```python
from build123d import *

# Parameters (mm, degrees)
SKETCH1_R      = 3.3274
EXTRUDE1_DEPTH = 152.4


with BuildPart() as part:
    # Sketch1 → Extrude1 (new body)
    with BuildSketch(Plane.XY):
        with BuildLine():
            Line((-10.022898969, 12.91475973), (-5.252158105, 8.144007132))
            ThreePointArc((-5.252158105, 8.144007132), (-3.715177372, 7.117027388), (-1.902183975, 6.7564))
            Line((-1.902183975, 6.7564), (1.902183975, 6.7564))
            ThreePointArc((1.902183975, 6.7564), (3.715177372, 7.117027388), (5.252158105, 8.144007132))
            Line((5.252158105, 8.144007132), (10.022898969, 12.91475973))
            ThreePointArc((10.022898969, 12.91475973), (10.218362387, 13.207291992), (10.287, 13.552357131))
            Line((10.287, 13.552357131), (10.287, 14.0843))
            ThreePointArc((10.287, 14.0843), (10.022898185, 14.721898185), (9.3853, 14.986))
            Line((9.3853, 14.986), (5.617617549, 14.986))
            ThreePointArc((5.617617549, 14.986), (4.519044045, 15.441044045), (4.064, 16.539617549))
            Line((4.064, 16.539617549), (4.064, 17.496382451))
            ThreePointArc((4.064, 17.496382451), (4.519044045, 18.594955955), (5.617617549, 19.05))
            Line((5.617617549, 19.05), (7.974178704, 19.05))
            ThreePointArc((7.974178704, 19.05), (8.736178704, 18.288), (9.498178704, 19.05))
            Line((9.498178704, 19.05), (14.327719207, 19.05))
            ThreePointArc((14.327719207, 19.05), (15.087603123, 18.231251131), (15.847487039, 19.05))
            ThreePointArc((15.847487039, 19.05), (18.120176289, 18.120192083), (19.05, 15.847509295))
            ThreePointArc((19.05, 15.847509295), (18.231250992, 15.08762539), (19.05, 14.327741484))
            Line((19.05, 14.327741484), (19.05, 9.496091471))
            ThreePointArc((19.05, 9.496091471), (18.231250992, 8.736207565), (19.05, 7.97632366))
            Line((19.05, 7.97632366), (19.05, 5.617617549))
            ThreePointArc((19.05, 5.617617549), (18.594955955, 4.519044045), (17.496382451, 4.064))
            Line((17.496382451, 4.064), (16.539617549, 4.064))
            ThreePointArc((16.539617549, 4.064), (15.441044045, 4.519044045), (14.986, 5.617617549))
            Line((14.986, 5.617617549), (14.986, 9.385342516))
            ThreePointArc((14.986, 9.385342516), (14.721898185, 10.022940701), (14.0843, 10.287042516))
            Line((14.0843, 10.287042516), (13.516042086, 10.287042516))
            ThreePointArc((13.516042086, 10.287042516), (13.170975923, 10.218404478), (12.878443117, 10.022939917))
            Line((12.878443117, 10.022939917), (8.14758008, 5.292065243))
            ThreePointArc((8.14758008, 5.292065243), (7.117955879, 3.751120653), (6.7564, 1.933453584))
            Line((6.7564, 1.933453584), (6.7564, -1.933453584))
            ThreePointArc((6.7564, -1.933453584), (7.117955879, -3.751120653), (8.14758008, -5.292065243))
            Line((8.14758008, -5.292065243), (12.878443117, -10.022939917))
            ThreePointArc((12.878443117, -10.022939917), (13.170975923, -10.218404478), (13.516042086, -10.287042516))
            Line((13.516042086, -10.287042516), (14.0843, -10.287042516))
            ThreePointArc((14.0843, -10.287042516), (14.721898185, -10.022940701), (14.986, -9.385342516))
            Line((14.986, -9.385342516), (14.986, -5.617617549))
            ThreePointArc((14.986, -5.617617549), (15.441044045, -4.519044045), (16.539617549, -4.064))
            Line((16.539617549, -4.064), (17.496382451, -4.064))
            ThreePointArc((17.496382451, -4.064), (18.594955955, -4.519044045), (19.05, -5.617617549))
            Line((19.05, -5.617617549), (19.05, -7.976318491))
            ThreePointArc((19.05, -7.976318491), (18.231250992, -8.736202396), (19.05, -9.496086302))
            Line((19.05, -9.496086302), (19.05, -14.32774291))
            ThreePointArc((19.05, -14.32774291), (18.231250992, -15.087626816), (19.05, -15.847510721))
            ThreePointArc((19.05, -15.847510721), (18.120175716, -18.120192644), (15.847486868, -19.05))
            ThreePointArc((15.847486868, -19.05), (15.087602952, -18.231251131), (14.327719036, -19.05))
            Line((14.327719036, -19.05), (9.496062448, -19.05))
            ThreePointArc((9.496062448, -19.05), (8.736178532, -18.231251131), (7.976294616, -19.05))
            Line((7.976294616, -19.05), (5.617617549, -19.05))
            ThreePointArc((5.617617549, -19.05), (4.519044045, -18.594955955), (4.064, -17.496382451))
            Line((4.064, -17.496382451), (4.064, -16.539617549))
            ThreePointArc((4.064, -16.539617549), (4.519044045, -15.441044045), (5.617617549, -14.986))
            Line((5.617617549, -14.986), (9.3853, -14.986))
            ThreePointArc((9.3853, -14.986), (10.022898185, -14.721898185), (10.287, -14.0843))
            Line((10.287, -14.0843), (10.287, -13.552357131))
            ThreePointArc((10.287, -13.552357131), (10.218362387, -13.207291992), (10.022898969, -12.91475973))
            Line((10.022898969, -12.91475973), (5.252158105, -8.144007132))
            ThreePointArc((5.252158105, -8.144007132), (3.715177372, -7.117027388), (1.902183975, -6.7564))
            Line((1.902183975, -6.7564), (-1.902183975, -6.7564))
            ThreePointArc((-1.902183975, -6.7564), (-3.715177372, -7.117027388), (-5.252158105, -8.144007132))
            Line((-5.252158105, -8.144007132), (-10.022898969, -12.91475973))
            ThreePointArc((-10.022898969, -12.91475973), (-10.218362387, -13.207291992), (-10.287, -13.552357131))
            Line((-10.287, -13.552357131), (-10.287, -14.0843))
            ThreePointArc((-10.287, -14.0843), (-10.022898185, -14.721898185), (-9.3853, -14.986))
            Line((-9.3853, -14.986), (-5.617617549, -14.986))
            ThreePointArc((-5.617617549, -14.986), (-4.519044045, -15.441044045), (-4.064, -16.539617549))
            Line((-4.064, -16.539617549), (-4.064, -17.496382451))
            ThreePointArc((-4.064, -17.496382451), (-4.519044045, -18.594955955), (-5.617617549, -19.05))
            Line((-5.617617549, -19.05), (-7.976294616, -19.05))
            ThreePointArc((-7.976294616, -19.05), (-8.736178532, -18.231251131), (-9.496062448, -19.05))
            Line((-9.496062448, -19.05), (-14.327719036, -19.05))
            ThreePointArc((-14.327719036, -19.05), (-15.087602952, -18.231251131), (-15.847486868, -19.05))
            ThreePointArc((-15.847486868, -19.05), (-18.120175716, -18.120192644), (-19.05, -15.847510721))
            ThreePointArc((-19.05, -15.847510721), (-18.231250992, -15.087626816), (-19.05, -14.32774291))
            Line((-19.05, -14.32774291), (-19.05, -9.496086302))
            ThreePointArc((-19.05, -9.496086302), (-18.231250992, -8.736202396), (-19.05, -7.976318491))
            Line((-19.05, -7.976318491), (-19.05, -5.617617549))
            ThreePointArc((-19.05, -5.617617549), (-18.594955955, -4.519044045), (-17.496382451, -4.064))
            Line((-17.496382451, -4.064), (-16.539617549, -4.064))
            ThreePointArc((-16.539617549, -4.064), (-15.441044045, -4.519044045), (-14.986, -5.617617549))
            Line((-14.986, -5.617617549), (-14.986, -9.385342516))
            ThreePointArc((-14.986, -9.385342516), (-14.721898185, -10.022940701), (-14.0843, -10.287042516))
            Line((-14.0843, -10.287042516), (-13.516042086, -10.287042516))
            ThreePointArc((-13.516042086, -10.287042516), (-13.170975923, -10.218404478), (-12.878443117, -10.022939917))
            Line((-12.878443117, -10.022939917), (-8.14758008, -5.292065243))
            ThreePointArc((-8.14758008, -5.292065243), (-7.117955879, -3.751120653), (-6.7564, -1.933453584))
            Line((-6.7564, -1.933453584), (-6.7564, 1.933453584))
            ThreePointArc((-6.7564, 1.933453584), (-7.117955879, 3.751120653), (-8.14758008, 5.292065243))
            Line((-8.14758008, 5.292065243), (-12.878443117, 10.022939917))
            ThreePointArc((-12.878443117, 10.022939917), (-13.170975923, 10.218404478), (-13.516042086, 10.287042516))
            Line((-13.516042086, 10.287042516), (-14.0843, 10.287042516))
            ThreePointArc((-14.0843, 10.287042516), (-14.721898185, 10.022940701), (-14.986, 9.385342516))
            Line((-14.986, 9.385342516), (-14.986, 5.617617549))
            ThreePointArc((-14.986, 5.617617549), (-15.441044045, 4.519044045), (-16.539617549, 4.064))
            Line((-16.539617549, 4.064), (-17.496382451, 4.064))
            ThreePointArc((-17.496382451, 4.064), (-18.594955955, 4.519044045), (-19.05, 5.617617549))
            Line((-19.05, 5.617617549), (-19.05, 7.97632366))
            ThreePointArc((-19.05, 7.97632366), (-18.231250992, 8.736207565), (-19.05, 9.496091471))
            Line((-19.05, 9.496091471), (-19.05, 14.327741484))
            ThreePointArc((-19.05, 14.327741484), (-18.231250992, 15.08762539), (-19.05, 15.847509295))
            ThreePointArc((-19.05, 15.847509295), (-18.120176289, 18.120192083), (-15.847487039, 19.05))
            ThreePointArc((-15.847487039, 19.05), (-15.087603123, 18.231251131), (-14.327719207, 19.05))
            Line((-14.327719207, 19.05), (-9.498178704, 19.05))
            ThreePointArc((-9.498178704, 19.05), (-8.736178704, 18.288), (-7.974178704, 19.05))
            Line((-7.974178704, 19.05), (-5.617617549, 19.05))
            ThreePointArc((-5.617617549, 19.05), (-4.519044045, 18.594955955), (-4.064, 17.496382451))
            Line((-4.064, 17.496382451), (-4.064, 16.539617549))
            ThreePointArc((-4.064, 16.539617549), (-4.519044045, 15.441044045), (-5.617617549, 14.986))
            Line((-5.617617549, 14.986), (-9.3853, 14.986))
            ThreePointArc((-9.3853, 14.986), (-10.022898185, 14.721898185), (-10.287, 14.0843))
            Line((-10.287, 14.0843), (-10.287, 13.552357131))
            ThreePointArc((-10.287, 13.552357131), (-10.218362387, 13.207291992), (-10.022898969, 12.91475973))
        make_face()
        Circle(SKETCH1_R, mode=Mode.SUBTRACT)
    extrude(amount=-EXTRUDE1_DEPTH)


solid = part.part
```
Verification items for the finished model (mm, model axes). A direction names the side the tool comes from. Give positions to 0.01 mm unless a question says otherwise; leave off trailing zeros. Order: outer loops, then holes, each group sorted by start corner. A loop starts at its lowest first (then second) coordinate and runs counter-clockwise, first axis right, second up. Notation, with made-up numbers: M 27.5,-9 L 53.5,-9 A22 ccw 53.5,2 Z; hole C 62,27 d11. An arc over 180 degrees is marked long. Answer in a Markdown table with one row per item. Add a question column.
Item 1: Mould release check, pull along X, two halves, no side actions. Record for faces 4 (the flat face through (12, -19.05, -75)), 5 (the flat face through (-14.986, 8, -75)): released by +X, released by -X, zero draft, split by the parting line, or undercut.
Item 2: Scan lines: probe 1 along Y at (x, z) = (-6.5, -37); probe 2 along Y at (x, z) = (0, -88); probe 3 along Y at (x, z) = (-14, -71). Record each from-to range of solid material in increasing order. Write a range as from..to.
Item 3: Section check A-A, the plane y = 0. Enter the section's corners in (x, z).
Item 4: Gauge pin test, flat ends, axial feed: pin 1 (1 mm diameter, centred on y = 3.5, z = -111.5, fed in from -X); pin 2 (0.8 mm diameter, centred on y = 17, z = -41.5, fed in from +X); pin 3 (1 mm diameter, centred on y = 2, z = -89, fed in from +X). Record the tip position at first contact, or that the pin passes through.
Item 5: Tool access check on faces 1 (the flat face through (7.604, 10.496, -75.133)), 2 (the flat face through (0, -6.756, -75)), 3 (the flat face through (5, 0, -152.4)). Record the directions out of +Z, -Z, +X, -X, +Y, -Y that give a thin tool (end or side, any length) a straight path to the whole face; none if there is none.
Filled sheet:
| question | item | result |
|---|---|---|
| 1 | face 4 | zero draft |
| 1 | face 5 | undercut |
| 2 | probe 1 | y = -19.05..-14.99, -9.39..9.39, 14.99..19.05 |
| 2 | probe 2 | y = -6.76..-3.33, 3.33..6.76 |
| 2 | probe 3 | y = -19.05..-10.29, 10.29..19.05 |
| 3 | outline | M -6.76,-152.4 L -3.33,-152.4 L -3.33,0 L -6.76,0 Z; M 3.33,-152.4 L 6.76,-152.4 L 6.76,0 L 3.33,0 Z |
| 4 | pin 1 | stops at x = -7.23 |
| 4 | pin 2 | stops at x = 18.97 |
| 4 | pin 3 | stops at x = 6.79 |
| 5 | face 1 | +Z, -Z |
| 5 | face 2 | +Z, -Z, -Y |
| 5 | face 3 | -Z, +X, -X, +Y, -Y |
